from build123d import *

# Parameters (mm, degrees)
F1_DEPTH = 3
F2_DEPTH = 20
F3_R     = 15


with BuildPart() as f1:
    # F0 (on Top) → F1 (new body)
    with BuildSketch(Plane.XY):
        Polygon((-84.4418774851, 68.0992258621), (-63.2286740495, 46.8860224265), (56.7713259505, 46.8860224265), align=None)
        Polygon((-63.2286740495, -73.1139775735), (-63.2286740495, 46.8860224265), (-84.4418774851, 68.0992258621), align=None)
        Polygon((-4.9964410025, -11.3462106205), (-58.2286740495, 41.8860224265), (-58.2286740495, -64.5784436676), align=None)
        with BuildLine():
            Line((48.2357920445, 41.8860224265), (-58.2286740495, 41.8860224265))
            add(Edge.make_bspline(
                [(-58.2286740495, 41.8860224265), (-27.8640476191, 22.2185579574), (-7.5944812554, 9.133690918), (6.3497696181, 0)],
                knots=[0, 0, 0, 0, 0.2321080347, 0.2321080347, 0.2321080347, 0.2321080347], degree=3))
            Line((6.3497696181, 0), (48.2357920445, 41.8860224265))
        make_face()
        Polygon((56.7713259505, 46.8860224265), (-63.2286740495, 46.8860224265), (-58.2286740495, 41.8860224265), (48.2357920445, 41.8860224265), (51.7713259505, 41.8860224265), (56.7713259505, 41.8860224265), align=None)
        Polygon((-58.2286740495, 41.8860224265), (-63.2286740495, 46.8860224265), (-63.2286740495, -73.1139775735), (-58.2286740495, -73.1139775735), (-58.2286740495, -68.1139775735), (-58.2286740495, -64.5784436676), align=None)
        Polygon((-1.4609070965, -14.8817445265), (-4.9964410025, -11.3462106205), (-58.2286740495, -64.5784436676), (-58.2286740495, -68.1139775735), (-54.6931401436, -68.1139775735), align=None)
        Polygon((51.7713259505, -68.1139775735), (-1.4609070965, -14.8817445265), (-54.6931401436, -68.1139775735), align=None)
        Polygon((-58.2286740495, -68.1139775735), (-58.2286740495, -73.1139775735), (56.7713259505, -73.1139775735), (51.7713259505, -68.1139775735), (-54.6931401436, -68.1139775735), align=None)
        Polygon((56.7713259505, -73.1139775735), (56.7713259505, 41.8860224265), (51.7713259505, 41.8860224265), (51.7713259505, 38.3504885206), (51.7713259505, -68.1139775735), align=None)
        with BuildLine():
            Line((51.7713259505, 38.3504885206), (10.6181651037, -2.8026723262))
            add(Edge.make_bspline(
                [(10.6181651037, -2.8026723262), (30.4463258159, -15.8579047438), (41.1308559966, -24.0461336089), (51.7713259505, -36.9598713142), (51.7713259505, -68.1139775735)],
                knots=[0.2569737781, 0.2569737781, 0.2569737781, 0.2569737781, 0.6213011396, 1, 1, 1, 1], degree=3))
            Line((51.7713259505, -68.1139775735), (51.7713259505, 38.3504885206))
        make_face()
        with BuildLine():
            Line((51.7713259505, 41.8860224265), (48.2357920445, 41.8860224265))
            Line((48.2357920445, 41.8860224265), (6.3497696181, 0))
            add(Edge.make_bspline(
                [(6.3497696181, 0), (7.8436177985, -0.9784926908), (9.2648713079, -1.9116383422), (10.6181651037, -2.8026723262)],
                knots=[0.2321080347, 0.2321080347, 0.2321080347, 0.2321080347, 0.2569737781, 0.2569737781, 0.2569737781, 0.2569737781], degree=3))
            Line((10.6181651037, -2.8026723262), (51.7713259505, 38.3504885206))
            Line((51.7713259505, 38.3504885206), (51.7713259505, 41.8860224265))
        make_face()
    extrude(amount=F1_DEPTH)

    # F0 (on Top) → F2 (join)
    with BuildSketch(Plane.XY):
        Polygon((56.7713259505, 46.8860224265), (-63.2286740495, 46.8860224265), (-58.2286740495, 41.8860224265), (48.2357920445, 41.8860224265), (51.7713259505, 41.8860224265), (56.7713259505, 41.8860224265), align=None)
        Polygon((-58.2286740495, 41.8860224265), (-63.2286740495, 46.8860224265), (-63.2286740495, -73.1139775735), (-58.2286740495, -73.1139775735), (-58.2286740495, -68.1139775735), (-58.2286740495, -64.5784436676), align=None)
    extrude(amount=F2_DEPTH)

    # F3
    f3_edges = [f1.edges().sort_by_distance(p)[0] for p in [
        (-60.728674, -73.113978, 20),
        (56.771326, 44.386022, 20),
        (-84.441877, 68.099226, 1.5),
    ]]
    fillet(f3_edges, radius=F3_R)


solid = f1.part
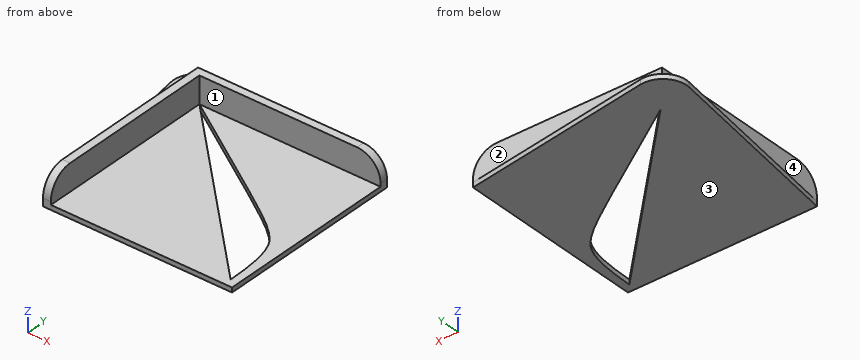
The listing builds one solid part. Answer for the finished solid, in the listing's coordinates (mm). Face numbers are marked on the shaded views. A direction names the side the tool comes from. Round coordinates to 2 decimals unless told otherwise and drop trailing zeros. Order: outer loops, then holes, each group sorted by start corner. A loop starts at its lowest first (then second) coordinate and runs counter-clockwise, first axis right, second up. Notation, with made-up numbers: (-18, -34) -> (34, -34) arc R22 ccw to (34, 3) -> close; hole circle Ø4 at (-6, 75). An arc over 180 degrees is marked (long way). Write each question's results on one line, items separated by ' | '. Start each with the question number.
Q1. Straight lines are drawn through the part: probe 1 along X at (y, z) = (39.5, 4); probe 2 along Z at (x, y) = (-0.5, -45); probe 3 along Y at (x, z) = (13, 3.25). For each, find the intervals that lie inside material, in ascending order. Write a range as from..to.
Q2. Each of these flat-tipped pins is pushed along its axis until it touches: pin 1 (2 mm diameter, centred on x = 24.5, y = -45.5, fed in from +Z); pin 2 (1 mm diameter, centred on x = -35.5, z = 6.5, fed in from +Y); pin 3 (8.5 mm diameter, centred on x = -7, z = 11.5, fed in from -Y). Where does it stop, or does it pass through?
Q3. Which of the six approach directions +Z, -Z, +X, -X, +Y, -Y give full straight-line access (tool end or side, diameter ignored) to the marked faces 1, 2, 3 and 4?
Q4. Find section A-A (z = 12). Determine the outline of the cut face in (x, y), then the cut area to 3 significant figures.
Q5. Find section B-B (x = -60.5). Determine the outline of the cut face in (y, z), then the cut area to 3 significant figures.
Worked answers:
1) probe 1: x = -63.23..-58.23 | probe 2: z = 0..3 | probe 3: y = 41.89..46.89
2) pin 1: stops at z = 3 | pin 2: stops at y = 46.89 | pin 3: stops at y = 41.89
3) face 1: +Z, +X, -Y | face 2: +Z, +X, -X, +Y | face 3: -Z, +X, -X, +Y, -Y | face 4: +Z, -X, +Y, -Y
4) outline: (-63.23, -71.38) -> (-58.23, -71.38) -> (-58.23, 41.89) -> (55.04, 41.89) -> (55.04, 46.89) -> (-63.23, 46.89) -> close | area: 1,160 mm2
5) outline: (-73.11, 0) -> (64.5, 0) -> (64.5, 3) -> (46.89, 3) -> (46.89, 20) -> (-58.11, 20) arc R15 ccw to (-73.11, 5) -> close | area: 2,400 mm2
